Read the model definition and answer for the solid it produces. Units are mm, in the model's axes. A direction names the side the tool comes from. Coordinates: 2 decimals unless noted, no trailing zeros. Loops run counter-clockwise (first coordinate to the right, second up) from the corner with the lowest first, then second, coordinate; pieces in that order, holes last. Notation, with made-up numbers: (57.5, 5) -> (110.5, 5) arc R22 cw to (110.5, 36) -> close; hole circle Ø7 at (9, 20). An arc over 180 degrees is marked (long way). Answer in a Markdown table with one row per item.
```python
from build123d import *

# Parameters (mm, degrees)
BOSS_EXTRUDE2_DEPTH   = 3.24
BOSS_EXTRUDE2_2_DEPTH = 3.24
SKETCH1_9_W           = 38.3
SKETCH1_9_H           = 20
BOSS_EXTRUDE3_DEPTH   = 13.04
SKETCH2_R             = 4.04
BOSS_EXTRUDE4_DEPTH   = 5.1
SKETCH1_10_W          = 38.3
SKETCH1_10_H          = 20
BOSS_EXTRUDE7_DEPTH   = 16.74
SKETCH5_W             = 38.3
SKETCH5_H             = 20
BOSS_EXTRUDE8_DEPTH   = 11.5
FILLET1_R             = 2.5
FILLET2_R             = 0.5
SKETCH6_R             = 2.03
CUT_EXTRUDE1_DEPTH    = 1.66


with BuildPart() as part:
    # Sketch1 → Boss-Extrude2 (new body)
    with BuildSketch(Plane(origin=(0, 0, 0), x_dir=(1, 0, 0), z_dir=(0, 1, 0))):
        with BuildLine():
            Line((-19.15, -10), (-19.15, 10))
            Line((-19.15, 10), (-24.75, 10))
            ThreePointArc((-24.75, 10), (-26.517766953, 9.267766953), (-27.25, 7.5))
            Line((-27.25, 7.5), (-27.25, 6))
            ThreePointArc((-27.25, 6), (-23.175424329, 5), (-27.25, 4))
            Line((-27.25, 4), (-27.25, -4))
            ThreePointArc((-27.25, -4), (-23.175424329, -5), (-27.25, -6))
            Line((-27.25, -6), (-27.25, -7.5))
            ThreePointArc((-27.25, -7.5), (-26.517766953, -9.267766953), (-24.75, -10))
            Line((-24.75, -10), (-19.15, -10))
        make_face()
    extrude(amount=BOSS_EXTRUDE2_DEPTH)



with BuildPart() as body_2:
    # Sketch1 → Boss-Extrude2 2 (new body)
    with BuildSketch(Plane(origin=(0, 0, 0), x_dir=(1, 0, 0), z_dir=(0, 1, 0))):
        with BuildLine():
            Line((24.75, 10), (19.15, 10))
            Line((19.15, 10), (19.15, -10))
            Line((19.15, -10), (24.75, -10))
            ThreePointArc((24.75, -10), (26.517766953, -9.267766953), (27.25, -7.5))
            Line((27.25, -7.5), (27.25, -6))
            ThreePointArc((27.25, -6), (23.175424329, -5), (27.25, -4))
            Line((27.25, -4), (27.25, 4))
            ThreePointArc((27.25, 4), (23.175424329, 5), (27.25, 6))
            Line((27.25, 6), (27.25, 7.5))
            ThreePointArc((27.25, 7.5), (26.517766953, 9.267766953), (24.75, 10))
        make_face()
    extrude(amount=BOSS_EXTRUDE2_2_DEPTH)


with BuildPart() as part_1:
    add(part.part)

    add(body_2.part)  # Boss-Extrude3 merges body 2
    # Sketch1<9> → Boss-Extrude3 (add)
    with BuildSketch(Plane(origin=(0, 0, 0), x_dir=(1, 0, 0), z_dir=(0, 1, 0))):
        Rectangle(SKETCH1_9_W, SKETCH1_9_H)
    extrude(amount=BOSS_EXTRUDE3_DEPTH)

    # Sketch2 → Boss-Extrude4 (add)
    with BuildSketch(Plane(origin=(0, 13.04, 0), x_dir=(1, 0, 0), z_dir=(0, 1, 0))):
        with Locations(Location((9.32, 0, 0), (0, 0, 270))):
            Circle(SKETCH2_R)
    extrude(amount=BOSS_EXTRUDE4_DEPTH)

    # Sketch1<10> → Boss-Extrude7 (add)
    with BuildSketch(Plane(origin=(0, 0, 0), x_dir=(1, 0, 0), z_dir=(0, 1, 0))):
        Rectangle(SKETCH1_10_W, SKETCH1_10_H)
    extrude(amount=-BOSS_EXTRUDE7_DEPTH)

    # Sketch5 → Boss-Extrude8 (add)
    with BuildSketch(Plane.XZ.offset(16.74)):
        Rectangle(SKETCH5_W, SKETCH5_H)
    extrude(amount=BOSS_EXTRUDE8_DEPTH)

    # Fillet1
    fillet1_edges = [part_1.edges().sort_by_distance(p)[0] for p in [
        (19.15, 13.04, 0),
        (0, 13.04, -10),
        (-19.15, 13.04, 0),
        (0, 13.04, 10),
        (9.32, 13.04, -4.04),
    ]]
    fillet(fillet1_edges, radius=FILLET1_R)

    # Fillet2
    fillet2_edges = [part_1.edges().sort_by_distance(p)[0] for p in [
        (-19.15, -28.24, 0),
        (0, -28.24, -10),
        (19.15, -28.24, 0),
        (0, -28.24, 10),
    ]]
    fillet(fillet2_edges, radius=FILLET2_R)

    # Sketch6 → Cut-Extrude1 (cut)
    with BuildSketch(Plane.XZ.offset(28.24)):
        with Locations((-16.22, 7.07)):
            Circle(SKETCH6_R)
        with BuildLine():
            Line((-18.65, 9.5), (-18.65, 5.04))
            Line((-18.65, 5.04), (-16.22, 5.04))
            ThreePointArc((-16.22, 5.04), (-17.655426766, 8.505426766), (-14.19, 7.07))
            Line((-14.19, 7.07), (-14.19, 9.5))
            Line((-14.19, 9.5), (-18.65, 9.5))
        make_face()
        with Locations((-16.22, -7.07)):
            Circle(SKETCH6_R)
        with BuildLine():
            Line((-16.22, -5.04), (-18.65, -5.04))
            Line((-18.65, -5.04), (-18.65, -9.5))
            Line((-18.65, -9.5), (-14.19, -9.5))
            Line((-14.19, -9.5), (-14.19, -7.07))
            ThreePointArc((-14.19, -7.07), (-17.655426766, -8.505426766), (-16.22, -5.04))
        make_face()
        with Locations((16.22, 6.97)):
            Circle(SKETCH6_R)
        with BuildLine():
            Line((18.65, 9.5), (14.19, 9.5))
            Line((14.19, 9.5), (14.19, 6.97))
            ThreePointArc((14.19, 6.97), (16.22, 9), (18.25, 6.97))
            ThreePointArc((18.25, 6.97), (17.655426766, 5.534573234), (16.22, 4.94))
            Line((16.22, 4.94), (18.65, 4.94))
            Line((18.65, 4.94), (18.65, 9.5))
        make_face()
        with Locations((16.22, -7.07)):
            Circle(SKETCH6_R)
        with BuildLine():
            Line((14.19, -7.07), (14.19, -9.5))
            Line((14.19, -9.5), (18.65, -9.5))
            Line((18.65, -9.5), (18.65, -5.04))
            Line((18.65, -5.04), (16.22, -5.04))
            ThreePointArc((16.22, -5.04), (17.655426766, -5.634573234), (18.25, -7.07))
            ThreePointArc((18.25, -7.07), (16.22, -9.1), (14.19, -7.07))
        make_face()
    extrude(amount=-CUT_EXTRUDE1_DEPTH, mode=Mode.SUBTRACT)


solid = part_1.part
```
1. A cutting plane is placed at D-D on x = -2.5. Give the vertices of the cut face in (y, z).
A:
| item | result |
|---|---|
| outline | (-28.24, -9.5) arc R0.5 ccw to (-27.74, -10) -> (10.54, -10) arc R2.5 ccw to (13.04, -7.5) -> (13.04, 7.5) arc R2.5 ccw to (10.54, 10) -> (-27.74, 10) arc R0.5 ccw to (-28.24, 9.5) -> close |
2. A cutting plane is placed at B-B on z = 0. Give the vertices of the cut face in (x, y).
A:
| item | result |
|---|---|
| outline | (-27.25, 0) -> (-19.15, 0) -> (-19.15, -27.74) arc R0.5 ccw to (-18.65, -28.24) -> (18.65, -28.24) arc R0.5 ccw to (19.15, -27.74) -> (19.15, 0) -> (27.25, 0) -> (27.25, 3.24) -> (19.15, 3.24) -> (19.15, 10.54) arc R2.5 ccw to (16.65, 13.04) -> (15.86, 13.04) arc R2.5 cw to (13.36, 15.54) -> (13.36, 18.14) -> (5.28, 18.14) -> (5.28, 15.54) arc R2.5 cw to (2.78, 13.04) -> (-16.65, 13.04) arc R2.5 ccw to (-19.15, 10.54) -> (-19.15, 3.24) -> (-27.25, 3.24) -> close |
3. Find the intervals of material crossed by probe 1 along X at (y, z) = (0.75, -5); probe 2 along X at (y, z) = (9.5, -4); probe 3 along Y at (x, z) = (-5.5, -4.25), in increasing order.
A:
| item | result |
|---|---|
| probe 1 | x = -23.18 to 23.18 |
| probe 2 | x = -19.15 to 19.15 |
| probe 3 | y = -28.24 to 13.04 |
4. A cutting plane is placed at C-C on y = 4. Give the vertices of the cut face in (x, z), and give its area (3 significant figures).
A:
| item | result |
|---|---|
| outline | (-19.15, -10) -> (19.15, -10) -> (19.15, 10) -> (-19.15, 10) -> close |
| area | 766 mm2 |
5. A cutting plane is placed at A-A on x = 9.32. Give the vertices of the cut face in (y, z), and give its area (3 significant figures).
A:
| item | result |
|---|---|
| outline | (-28.24, -9.5) arc R0.5 ccw to (-27.74, -10) -> (10.54, -10) arc R2.5 ccw to (13.04, -7.5) -> (13.04, -6.54) arc R2.5 cw to (15.54, -4.04) -> (18.14, -4.04) -> (18.14, 4.04) -> (15.54, 4.04) arc R2.5 cw to (13.04, 6.54) -> (13.04, 7.5) arc R2.5 ccw to (10.54, 10) -> (-27.74, 10) arc R0.5 ccw to (-28.24, 9.5) -> close |
| area | 867 mm2 |
6. The mould has two halves that part along Z. Classify faces 6 (the flat face through (0, -8, 10)), 7 (the cylindrical face through (-14.8, -27.42, 5.62)), 8 (the cylindrical face through (18.398, 12.327, -0.14)), 9 (the flat face through (-17, -27, -5.04)): pulls with the +Z half, pulls with the -Z half, needs draft (parallel to the pull), parting line crosses it, or undercut.
A:
| item | result |
|---|---|
| face 6 | pulls with the +Z half |
| face 7 | undercut |
| face 8 | needs draft |
| face 9 | undercut |
7. Given pin 1 Ø9 at (x, z) = (22, -1.5) entering from +Y; pin 2 Ø4 at (x, z) = (-23.5, -1.5) entering from +Y; pin 3 Ø9 at (x, z) = (23.5, 3.5) entering from -Y, each flat-ended and moving along its own axis, determine where each tip first touches the part or whether it passes through.
A:
| item | result |
|---|---|
| pin 1 | stops at y = 12.89 |
| pin 2 | stops at y = 3.24 |
| pin 3 | stops at y = -28.1 |
8. A tool of negligible diameter and unlimited length cuts with its end or side. For faces 1 (the flat face through (-22, 0, 0)), 2 (the flat face through (19.15, -14, 0)), 3 (the flat face through (22, 3.24, 0)), 4 (the cylindrical face through (-14.77, -27.42, -5.65)), 5 (the flat face through (-19.15, 7, 0)), from which of +Z, -Z, +X, -X, +Y, -Y can it reach the whole face along a straight path? Write none if from no direction.
A:
| item | result |
|---|---|
| face 1 | +Z, -Z, -X, -Y |
| face 2 | +Z, -Z, +X, -Y |
| face 3 | +Z, -Z, +X, +Y |
| face 4 | -Y |
| face 5 | +Z, -Z, -X, +Y |
